Work out the finished part from the listing and answer in its coordinate system (mm). A direction names the side the tool comes from. Round coordinates to 2 decimals unless told otherwise and drop trailing zeros. One line per question, with ' | ' between items. Start each with the question number.
```python
from build123d import *

# Parameters (mm, degrees)
SKETCH1_R             = 9.525
SKETCH1_R_2           = 8.7122
BOSS_EXTRUDE1_DEPTH   = 1.5875
SKETCH1_R_3           = 7.95655
SKETCH1_R_4           = 7.14375
BOSS_EXTRUDE1_2_DEPTH = 1.5875
FILLET1_R             = 0.127
CHAMFER1_SIZE         = 0.127
SKETCH2_R             = 8.7122
SKETCH2_R_2           = 7.95655
BOSS_EXTRUDE2_DEPTH   = 1.4605


with BuildPart() as part:
    # Sketch1 → Boss-Extrude1 (new body, symmetric)
    with BuildSketch(Plane(origin=(0, 0, 0), x_dir=(1, 0, 0), z_dir=(0, 1, 0))):
        Circle(SKETCH1_R)
        Circle(SKETCH1_R_2, mode=Mode.SUBTRACT)
    extrude(amount=BOSS_EXTRUDE1_DEPTH, both=True)

    # Fillet1
    fillet1_edges = [part.edges().sort_by_distance(p)[0] for p in [
        (-9.525, -1.5875, 0),
        (-9.525, 1.5875, 0),
    ]]
    fillet(fillet1_edges, radius=FILLET1_R)



with BuildPart() as body_2:
    # Sketch1 → Boss-Extrude1 2 (new body, symmetric)
    with BuildSketch(Plane(origin=(0, 0, 0), x_dir=(1, 0, 0), z_dir=(0, 1, 0))):
        Circle(SKETCH1_R_3)
        Circle(SKETCH1_R_4, mode=Mode.SUBTRACT)
    extrude(amount=BOSS_EXTRUDE1_2_DEPTH, both=True)

    # Chamfer1
    chamfer1_edges = [body_2.edges().sort_by_distance(p)[0] for p in [
        (-7.14375, -1.5875, 0),
        (-7.14375, 1.5875, 0),
    ]]
    chamfer(chamfer1_edges, length=CHAMFER1_SIZE)


with BuildPart() as part_1:
    add(part.part)

    add(body_2.part)  # Boss-Extrude2 merges body 2
    # Sketch2 → Boss-Extrude2 (add, symmetric)
    with BuildSketch(Plane(origin=(0, 0, 0), x_dir=(1, 0, 0), z_dir=(0, 1, 0))):
        Circle(SKETCH2_R)
        Circle(SKETCH2_R_2, mode=Mode.SUBTRACT)
    extrude(amount=BOSS_EXTRUDE2_DEPTH, both=True)


solid = part_1.part
```
(1) Given pin 1 Ø6 at (x, z) = (3.5, 4) entering from -Y, flat-ended and moving along its own axis, determine where the tip first touches the part or whether it passes through.
(2) Consider L1, parallel to Z at x = 0, y = 1.55; L2, parallel to X at y = 0.7, z = 0 (3 decimals); L3, parallel to X at y = -1.5, z = 0. Determine where each line is inside the solid, lowest interval first.
(3) The mould has two halves that part along X. Classify faces 3 (the cylindrical face through (-7.559, 0.02, 5.796)), 4 (the flat face through (6, -1.588, 7)), 5 (the flat face through (3, -1.46, 8)), 6 (the cylindrical face through (-7.137, -0.02, -0.314)): +X half, -X half, draft (parallel to the pull), parting line (faces both ways), or undercut.
(4) For faces 1 (the flat face through (3, 1.46, 8)), 2 (the flat face through (6, 1.588, 7)), determine the directions among +Z, -Z, +X, -X, +Y, -Y from which every point of the face is accessible in a straight line to the end or side of a thin tool.
Returned:
1) pin 1: y = -1.59
2) L1: -9.49 to -8.71, -7.96 to -7.23, 7.23 to 7.96, 8.71 to 9.49 | L2: -9.525 to -7.144, 7.144 to 9.525 | L3: -9.52 to -8.71, -7.96 to -7.18, 7.18 to 7.96, 8.71 to 9.52
3) face 3: parting line | face 4: draft | face 5: undercut | face 6: undercut
4) face 1: +Y | face 2: +Z, -Z, +X, -X, +Y
